Drawing for the job (mm, zero at the part's lowest x, y, z). Coordinates: 2 decimals unless noted, no trailing zeros. Order: outer loops, then holes, each group sorted by start corner. A loop starts at its lowest first (then second) coordinate and runs counter-clockwise, first axis right, second up.
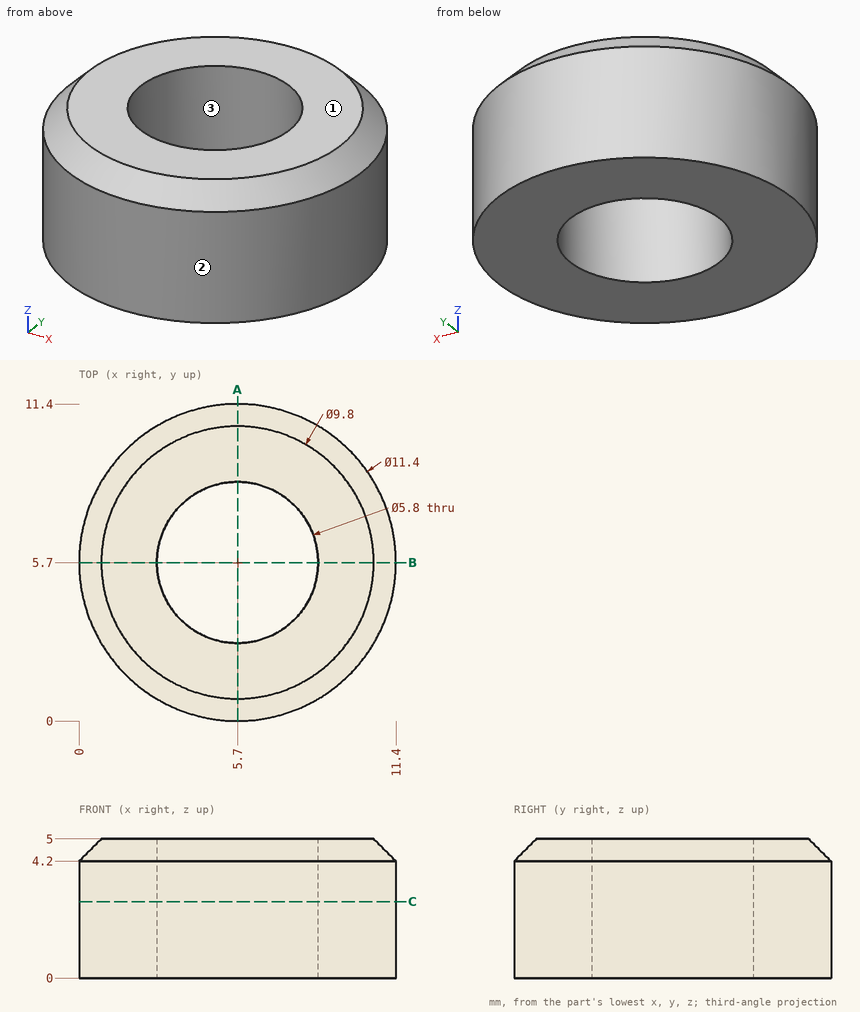
1) Two-plate mould, pull along Y, no slides. Class the marked faces 1, 2 and 3: released by +Y, released by -Y, zero draft, split by the parting line, or undercut.
2) Slice it at A-A (x = 5.7). List the corners of the cut face in (y, z), plus the area to 3 significant figures.
3) Pin check, flat tips, straight feed: P1, Ø1.5, axis at x = 7, z = 3, coming from the +Y side; P2, Ø4.5, axis at x = 5.7, y = 5.7, coming from the +Z side. Stop position of each tip, or through.
4) Drill centre lines: probe 1 along Y at (x, z) = (5.7, 1.5); probe 2 along X at (y, z) = (7.25, 1.5); probe 3 along X at (y, z) = (4, 1.5). Where is each one in solid material? Low to high.
5) Slice it at C-C (z = 2.75). List the corners of the cut face in (x, y).
Worked out:
1. face 1: zero draft
1. face 2: split by the parting line
1. face 3: undercut
2. outline: (0, 0) - (2.8, 0) - (2.8, 5) - (0.8, 5) - (0, 4.2) - close; (8.6, 0) - (11.4, 0) - (11.4, 4.2) - (10.6, 5) - (8.6, 5) - close
2. area: 27.4 mm2
3. P1: stops at y = 11.37
3. P2: passes through
4. probe 1: y = 0 to 2.8, 8.6 to 11.4
4. probe 2: x = 0.21 to 3.25, 8.15 to 11.19
4. probe 3: x = 0.26 to 3.35, 8.05 to 11.14
5. outline: circle Ø11.4 at (5.7, 5.7); hole circle Ø5.8 at (5.7, 5.7)
